from build123d import *

# Parameters (mm, degrees)
BODYSKE_R  = 1
BODY_DEPTH = 1.5


with BuildPart() as part:
    # BodySke → Body (new body)
    with BuildSketch(Plane.XY):
        with BuildLine():
            Line((3.225876843, -12.69660264), (2.477844243, -9.752450354))
            ThreePointArc((2.477844243, -9.752450354), (3.416111801, -7.362891432), (5.980158955, -7.489382725))
            ThreePointArc((5.980158955, -7.489382725), (7.701462242, -7.939845491), (9.193020908, -6.96976588))
            ThreePointArc((9.193020908, -6.96976588), (0, 10), (-9.193020908, -6.96976588))
            ThreePointArc((-9.193020908, -6.96976588), (-7.701462242, -7.939845491), (-5.980158955, -7.489382725))
            ThreePointArc((-5.980158955, -7.489382725), (-3.416111801, -7.362891432), (-2.477844243, -9.752450354))
            Line((-2.477844243, -9.752450354), (-3.225876843, -12.69660264))
            ThreePointArc((-3.225876843, -12.69660264), (0, 13.1), (3.225876843, -12.69660264))
        make_face()
        with Locations((4.610098122, -9.210700044)):
            Circle(BODYSKE_R, mode=Mode.SUBTRACT)
        with Locations((-4.610098122, -9.210700044)):
            Circle(BODYSKE_R, mode=Mode.SUBTRACT)
    extrude(amount=-BODY_DEPTH)


solid = part.part
Work out the finished part from the listing and answer in its coordinate system (mm). A direction names the side the tool comes from. Coordinates: 2 decimals unless noted, no trailing zeros. Write each loop counter-clockwise with the first axis right and the second up, starting at its lowest first coordinate (ties: lowest second). Pieces come first, ordered by that corner, then holes. Notation, with made-up numbers: (69, 71.25) - (84, 71.25) arc R26 ccw to (84, 108.25) - close; hole circle Ø4 at (-4.75, 54.25). An arc over 180 degrees is marked (long way). One line per question, with ' | ' between items.
1) Consider probe 1 along Y at (x, z) = (-4.5, -0.75); probe 2 along X at (y, z) = (-9, -0.15); probe 3 along Y at (x, z) = (7.5, -1). Determine where each line is inside the solid, lowest interval first. Write a range as [from, to].
Checks:
probe 1: [-12.3, -10.2], [-8.22, -7.01], [9.04, 12.3] | probe 2: [-9.52, -5.59], [-3.63, -2.42], [2.42, 3.63], [5.59, 9.52] | probe 3: [-10.74, -7.96], [7.04, 10.74]
2) Find section D-D, the plane x = 10.5. Determine the outline of the cut face in (y, z).
Checks:
outline: (-7.83, -1.5) - (-4.17, -1.5) - (-4.17, 0) - (-7.83, 0) - close; (2.22, -1.5) - (7.83, -1.5) - (7.83, 0) - (2.22, 0) - close
3) Find section B-B, the plane z = -0.8. Determine the outline of the cut face in (x, y).
Checks:
outline: (-9.19, -6.97) arc R10.97 cw (long way) to (9.19, -6.97) arc R2.2 cw to (5.98, -7.49) arc R2.2 ccw to (2.48, -9.75) - (3.23, -12.7) arc R13.1 ccw (long way) to (-3.23, -12.7) - (-2.48, -9.75) arc R2.2 ccw to (-5.98, -7.49) arc R2.2 cw to start; hole circle Ø2 at (-4.61, -9.21); hole circle Ø2 at (4.61, -9.21)
4) For faces 1 (the face through (-3.8, -7.4, 0)), 2 (the face through (-2.847, -11.204, -0.74)), determine the directions among +Z, -Z, +X, -X, +Y, -Y from which every point of the face is accessible in a straight line to the end or side of a thin tool.
Checks:
face 1: +Z, +X, -X, +Y, -Y | face 2: +Z, -Z, -Y
5) The mould has two halves that part along X. Classify faces 3 (the face through (-3.8, -7.4, -1.5)), 4 (the face through (3.61, -9.17, -0.74)), 5 (the face through (-0.53, 13.09, -0.74)): +X half, -X half, draft (parallel to the pull), parting line (faces both ways), or undercut.
Checks:
face 3: draft | face 4: undercut | face 5: parting line
6) A flat-ended cylindrical pin translates along its axis: P1, Ø1.8, axis at x = -4.61, y = -9.21, coming from the -Z side. Find the tip coordinate at first contact, or state that the pin passes through.
Checks:
P1: through
7) Find section A-A, the plane y = 9. Determine the outline of the cut face in (x, z), and give its area (3 significant figures).
Checks:
outline: (-9.52, -1.5) - (-4.58, -1.5) - (-4.58, 0) - (-9.52, 0) - close; (4.58, -1.5) - (9.52, -1.5) - (9.52, 0) - (4.58, 0) - close | area: 14.8 mm2
8) Find section C-C, the plane x = 4.75. Determine the outline of the cut face in (y, z).
Checks:
outline: (-12.21, -1.5) - (-10.2, -1.5) - (-10.2, 0) - (-12.21, 0) - close; (-8.22, -1.5) - (-7.02, -1.5) - (-7.02, 0) - (-8.22, 0) - close; (8.92, -1.5) - (12.21, -1.5) - (12.21, 0) - (8.92, 0) - close
